The listing builds one solid part. Answer for the finished solid, in the listing's coordinates (mm). A direction names the side the tool comes from. Give positions to 0.01 mm unless a question says otherwise; leave off trailing zeros. Loops run counter-clockwise (first coordinate to the right, second up) from the corner with the lowest first, then second, coordinate; pieces in that order, holes last.
Item 1: Section B-B, the plane y = 7.25 is taken. Give the vertices of the cut face in (x, z).
Item 2: A tool of negligible diameter and unlimited length cuts with its end or side. For faces 4 (the face through (-4.33, 10.9, -3.16)), 5 (the face through (-7.81, 6.38, -1.73)), from which of +Z, -Z, +X, -X, +Y, -Y can it reach the whole face along a straight path? Write none if from no direction.
Item 3: Section A-A, the plane x = 0 is taken. Give the vertices of the cut face in (y, z).
Item 4: Each of these flat-tipped pins is pushed along its axis until it touches: pin 1 Ø3 at (y, z) = (10, -5) entering from -X; pin 2 Ø3 at (x, y) = (-6, 7) entering from -Z; pin 3 Ø6 at (x, y) = (-4, 11) entering from -Z. Where does it stop, or does it pass through?
Item 5: Consider line 1 along Y through (x, z) = (-0.25, -7); line 2 along Z through (x, y) = (-5.5, 11.25). Determine where each line is inside the solid, lowest interval first.
Item 6: The mould has two halves that part along Y. Classify faces 1 (the face through (-2, 5.9, 4)), 2 (the face through (-7.81, 15.51, -1.73)), 3 (the face through (0.01, 10.9, -5.36)): pulls with the +Y half, pulls with the -Y half, needs draft (parallel to the pull), parting line crosses it, or undercut.
from build123d import *
from OCP.BRepFilletAPI import BRepFilletAPI_MakeChamfer

# Parameters (mm, degrees)
SKETCH_1_R               = 8
SKETCH_1_R_2             = 2.5
EXTRUDE_1_DEPTH          = 7.45
SKETCH_2_R               = 2.5
EXTRUDE_2_DEPTH          = 7
SKETCH_3_R               = 8
SKETCH_3_R_2             = 2.5
EXTRUDE_3_DEPTH          = 1.55
CUT_EXTRUDE_1_REACH      = 21.596
CUT_EXTRUDE_1_END_RADIUS = 8
SKETCH_4_R               = 1.25
CUT_EXTRUDE_2_REACH      = 21.596
CUT_EXTRUDE_2_END_RADIUS = 8
SKETCH_5_R               = 1.25
CHAMFER_1_SIZE           = 1
CHAMFER_1_SIZE2          = 0.577350269
ESBO_O1_R                = 8
CORTE_EXTRUS_O1_DEPTH    = 5.9
ESBO_O2_R                = 4
CORTE_EXTRUS_O2_DEPTH    = 10.1


with BuildPart() as part:
    # Эскиз1 → Бобышка-Вытянуть1 (new body)
    with BuildSketch(Plane(origin=(0, 0, 0), x_dir=(1, 0, 0), z_dir=(0, 1, 0))):
        with Locations(Location((0, 0, 0), (0, 0, 270))):
            Circle(SKETCH_1_R)
        with Locations(Location((0, 0, 0), (0, 0, 270))):
            Circle(SKETCH_1_R_2, mode=Mode.SUBTRACT)
    extrude(amount=EXTRUDE_1_DEPTH)

    # Эскиз2 → Бобышка-Вытянуть2 (add)
    with BuildSketch(Plane(origin=(0, 7.45, 0), x_dir=(1, 0, 0), z_dir=(0, 1, 0))):
        with BuildLine():
            ThreePointArc((-2.557469435, 5.549004423), (-2.773881953, 5.444049863), (-2.985996064, 5.3306592))
            ThreePointArc((-2.985996064, 5.3306592), (-3.059404709, 5.231014138), (-3.032930262, 5.110113057))
            ThreePointArc((-3.032930262, 5.110113057), (-3.150528952, 4.33633109), (-3.922779328, 4.463599867))
            ThreePointArc((-3.922779328, 4.463599867), (-4.029582035, 4.526139051), (-4.14703464, 4.487115298))
            ThreePointArc((-4.14703464, 4.487115298), (-4.320422433, 4.320422433), (-4.487115298, 4.14703464))
            ThreePointArc((-4.487115298, 4.14703464), (-4.526139051, 4.029582035), (-4.463599867, 3.922779328))
            ThreePointArc((-4.463599867, 3.922779328), (-4.33633109, 3.150528952), (-5.110113057, 3.032930262))
            ThreePointArc((-5.110113057, 3.032930262), (-5.231014138, 3.059404709), (-5.3306592, 2.985996064))
            ThreePointArc((-5.3306592, 2.985996064), (-5.444049863, 2.773881953), (-5.549004423, 2.557469435))
            ThreePointArc((-5.549004423, 2.557469435), (-5.549823367, 2.433706366), (-5.457341217, 2.351456627))
            ThreePointArc((-5.457341217, 2.351456627), (-5.097662927, 1.65633109), (-5.797233315, 1.305376312))
            ThreePointArc((-5.797233315, 1.305376312), (-5.92039813, 1.293194518), (-5.992481697, 1.19258673))
            ThreePointArc((-5.992481697, 1.19258673), (-6.034775761, 0.955814581), (-6.067718334, 0.717561302))
            ThreePointArc((-6.067718334, 0.717561302), (-6.030252304, 0.599602562), (-5.916879985, 0.549956967))
            ThreePointArc((-5.916879985, 0.549956967), (-5.36, 0), (-5.916879985, -0.549956967))
            ThreePointArc((-5.916879985, -0.549956967), (-6.030252304, -0.599602562), (-6.067718334, -0.717561302))
            ThreePointArc((-6.067718334, -0.717561302), (-6.034775761, -0.955814581), (-5.992481697, -1.19258673))
            ThreePointArc((-5.992481697, -1.19258673), (-5.92039813, -1.293194518), (-5.797233315, -1.305376312))
            ThreePointArc((-5.797233315, -1.305376312), (-5.097662927, -1.65633109), (-5.457341217, -2.351456627))
            ThreePointArc((-5.457341217, -2.351456627), (-5.549823367, -2.433706366), (-5.549004423, -2.557469435))
            ThreePointArc((-5.549004423, -2.557469435), (-5.444049863, -2.773881953), (-5.3306592, -2.985996064))
            ThreePointArc((-5.3306592, -2.985996064), (-5.231014138, -3.059404709), (-5.110113057, -3.032930262))
            ThreePointArc((-5.110113057, -3.032930262), (-4.33633109, -3.150528952), (-4.463599867, -3.922779328))
            ThreePointArc((-4.463599867, -3.922779328), (-4.526139051, -4.029582035), (-4.487115298, -4.14703464))
            ThreePointArc((-4.487115298, -4.14703464), (-4.320422433, -4.320422433), (-4.14703464, -4.487115298))
            ThreePointArc((-4.14703464, -4.487115298), (-4.029582035, -4.526139051), (-3.922779328, -4.463599867))
            ThreePointArc((-3.922779328, -4.463599867), (-3.150528952, -4.33633109), (-3.032930262, -5.110113057))
            ThreePointArc((-3.032930262, -5.110113057), (-3.059404709, -5.231014138), (-2.985996064, -5.3306592))
            ThreePointArc((-2.985996064, -5.3306592), (-2.773881953, -5.444049863), (-2.557469435, -5.549004423))
            ThreePointArc((-2.557469435, -5.549004423), (-2.433706366, -5.549823367), (-2.351456627, -5.457341217))
            ThreePointArc((-2.351456627, -5.457341217), (-1.65633109, -5.097662927), (-1.305376312, -5.797233315))
            ThreePointArc((-1.305376312, -5.797233315), (-1.293194518, -5.92039813), (-1.19258673, -5.992481697))
            ThreePointArc((-1.19258673, -5.992481697), (-0.955814581, -6.034775761), (-0.717561302, -6.067718334))
            ThreePointArc((-0.717561302, -6.067718334), (-0.599602562, -6.030252304), (-0.549956967, -5.916879985))
            ThreePointArc((-0.549956967, -5.916879985), (0, -5.36), (0.549956967, -5.916879985))
            ThreePointArc((0.549956967, -5.916879985), (0.599602562, -6.030252304), (0.717561302, -6.067718334))
            ThreePointArc((0.717561302, -6.067718334), (0.955814581, -6.034775761), (1.19258673, -5.992481697))
            ThreePointArc((1.19258673, -5.992481697), (1.293194518, -5.92039813), (1.305376312, -5.797233315))
            ThreePointArc((1.305376312, -5.797233315), (1.65633109, -5.097662927), (2.351456627, -5.457341217))
            ThreePointArc((2.351456627, -5.457341217), (2.433706366, -5.549823367), (2.557469435, -5.549004423))
            ThreePointArc((2.557469435, -5.549004423), (2.773881953, -5.444049863), (2.985996064, -5.3306592))
            ThreePointArc((2.985996064, -5.3306592), (3.059404709, -5.231014138), (3.032930262, -5.110113057))
            ThreePointArc((3.032930262, -5.110113057), (3.150528952, -4.33633109), (3.922779328, -4.463599867))
            ThreePointArc((3.922779328, -4.463599867), (4.029582035, -4.526139051), (4.14703464, -4.487115298))
            ThreePointArc((4.14703464, -4.487115298), (4.320422433, -4.320422433), (4.487115298, -4.14703464))
            ThreePointArc((4.487115298, -4.14703464), (4.526139051, -4.029582035), (4.463599867, -3.922779328))
            ThreePointArc((4.463599867, -3.922779328), (4.33633109, -3.150528952), (5.110113057, -3.032930262))
            ThreePointArc((5.110113057, -3.032930262), (5.231014138, -3.059404709), (5.3306592, -2.985996064))
            ThreePointArc((5.3306592, -2.985996064), (5.444049863, -2.773881953), (5.549004423, -2.557469435))
            ThreePointArc((5.549004423, -2.557469435), (5.549823367, -2.433706366), (5.457341217, -2.351456627))
            ThreePointArc((5.457341217, -2.351456627), (5.097662927, -1.65633109), (5.797233315, -1.305376312))
            ThreePointArc((5.797233315, -1.305376312), (5.92039813, -1.293194518), (5.992481697, -1.19258673))
            ThreePointArc((5.992481697, -1.19258673), (6.034775761, -0.955814581), (6.067718334, -0.717561302))
            ThreePointArc((6.067718334, -0.717561302), (6.030252304, -0.599602562), (5.916879985, -0.549956967))
            ThreePointArc((5.916879985, -0.549956967), (5.36, 0), (5.916879985, 0.549956967))
            ThreePointArc((5.916879985, 0.549956967), (6.030252304, 0.599602562), (6.067718334, 0.717561302))
            ThreePointArc((6.067718334, 0.717561302), (6.034775761, 0.955814581), (5.992481697, 1.19258673))
            ThreePointArc((5.992481697, 1.19258673), (5.92039813, 1.293194518), (5.797233315, 1.305376312))
            ThreePointArc((5.797233315, 1.305376312), (5.097662927, 1.65633109), (5.457341217, 2.351456627))
            ThreePointArc((5.457341217, 2.351456627), (5.549823367, 2.433706366), (5.549004423, 2.557469435))
            ThreePointArc((5.549004423, 2.557469435), (5.444049863, 2.773881953), (5.3306592, 2.985996064))
            ThreePointArc((5.3306592, 2.985996064), (5.231014138, 3.059404709), (5.110113057, 3.032930262))
            ThreePointArc((5.110113057, 3.032930262), (4.33633109, 3.150528952), (4.463599867, 3.922779328))
            ThreePointArc((4.463599867, 3.922779328), (4.526139051, 4.029582035), (4.487115298, 4.14703464))
            ThreePointArc((4.487115298, 4.14703464), (4.320422433, 4.320422433), (4.14703464, 4.487115298))
            ThreePointArc((4.14703464, 4.487115298), (4.029582035, 4.526139051), (3.922779328, 4.463599867))
            ThreePointArc((3.922779328, 4.463599867), (3.150528952, 4.33633109), (3.032930262, 5.110113057))
            ThreePointArc((3.032930262, 5.110113057), (3.059404709, 5.231014138), (2.985996064, 5.3306592))
            ThreePointArc((2.985996064, 5.3306592), (2.773881953, 5.444049863), (2.557469435, 5.549004423))
            ThreePointArc((2.557469435, 5.549004423), (2.433706366, 5.549823367), (2.351456627, 5.457341217))
            ThreePointArc((2.351456627, 5.457341217), (1.65633109, 5.097662927), (1.305376312, 5.797233315))
            ThreePointArc((1.305376312, 5.797233315), (1.293194518, 5.92039813), (1.19258673, 5.992481697))
            ThreePointArc((1.19258673, 5.992481697), (0.955814581, 6.034775761), (0.717561302, 6.067718334))
            ThreePointArc((0.717561302, 6.067718334), (0.599602562, 6.030252304), (0.549956967, 5.916879985))
            ThreePointArc((0.549956967, 5.916879985), (0, 5.36), (-0.549956967, 5.916879985))
            ThreePointArc((-0.549956967, 5.916879985), (-0.599602562, 6.030252304), (-0.717561302, 6.067718334))
            ThreePointArc((-0.717561302, 6.067718334), (-0.955814581, 6.034775761), (-1.19258673, 5.992481697))
            ThreePointArc((-1.19258673, 5.992481697), (-1.293194518, 5.92039813), (-1.305376312, 5.797233315))
            ThreePointArc((-1.305376312, 5.797233315), (-1.65633109, 5.097662927), (-2.351456627, 5.457341217))
            ThreePointArc((-2.351456627, 5.457341217), (-2.433706366, 5.549823367), (-2.557469435, 5.549004423))
        make_face()
        with Locations(Location((0, 0, 0), (0, 0, 270))):
            Circle(SKETCH_2_R, mode=Mode.SUBTRACT)
    extrude(amount=EXTRUDE_2_DEPTH)

    # Эскиз3 → Бобышка-Вытянуть3 (add)
    with BuildSketch(Plane(origin=(0, 14.45, 0), x_dir=(1, 0, 0), z_dir=(0, 1, 0))):
        with Locations(Location((0, 0, 0), (0, 0, 270))):
            Circle(SKETCH_3_R)
        with Locations(Location((0, 0, 0), (0, 0, 270))):
            Circle(SKETCH_3_R_2, mode=Mode.SUBTRACT)
    extrude(amount=EXTRUDE_3_DEPTH)

    # Вырез-Вытянуть1: up to this cylinder (the profile starts inside it)
    cut_extrude_1_end = Plane(origin=(0, 3.725, 0), z_dir=(0, -1, 0)) * Cylinder(CUT_EXTRUDE_1_END_RADIUS, 60.192, mode=Mode.PRIVATE)
    # Эскиз4 → Вырез-Вытянуть1 (cut, up to the surface)
    with BuildSketch(Plane.XY, mode=Mode.PRIVATE) as cut_extrude_1_sk1:
        with Locations(Location((0, 3.725, 0), (0, 0, 180))):
            Circle(SKETCH_4_R)
    cut_extrude_1_tool1 = extrude(cut_extrude_1_sk1.sketch, amount=CUT_EXTRUDE_1_REACH, mode=Mode.PRIVATE) & cut_extrude_1_end
    add(cut_extrude_1_tool1.solids().sort_by_distance((0, 3.725, 0))[0], mode=Mode.SUBTRACT)

    # Вырез-Вытянуть2: up to this cylinder (the profile starts inside it)
    cut_extrude_2_end = Plane(origin=(0, 3.725, 0), z_dir=(0, -1, 0)) * Cylinder(CUT_EXTRUDE_2_END_RADIUS, 60.192, mode=Mode.PRIVATE)
    # Эскиз5 → Вырез-Вытянуть2 (cut, up to the surface)
    with BuildSketch(Plane(origin=(0, 0, 0), x_dir=(0, 0, -1), z_dir=(1, 0, 0)), mode=Mode.PRIVATE) as cut_extrude_2_sk1:
        with Locations(Location((0, 3.725, 0), (0, 0, 180))):
            Circle(SKETCH_5_R)
    cut_extrude_2_tool1 = extrude(cut_extrude_2_sk1.sketch, amount=CUT_EXTRUDE_2_REACH, mode=Mode.PRIVATE) & cut_extrude_2_end
    add(cut_extrude_2_tool1.solids().sort_by_distance((0, 3.725, 0))[0], mode=Mode.SUBTRACT)

    # Фаска1: one chamfer whose edges measure the first distance from different faces: ONE call of the kernel's chamfer builder (chamfer() names one face for all edges)
    chamfer_1_edges_1 = [part.edges().sort_by_distance(p)[0] for p in [
        (0, 14.45, -8),
    ]]
    chamfer_1_side_1 = [part.faces().sort_by_distance(p)[0] for p in [
        (0, 14.45, -7.77372583),
    ]]
    chamfer_1_edges_2 = [part.edges().sort_by_distance(p)[0] for p in [
        (0, 7.45, -8),
    ]]
    chamfer_1_side_2 = [part.faces().sort_by_distance(p)[0] for p in [
        (0, 7.45, -7.77372583),
    ]]
    chamfer_1 = BRepFilletAPI_MakeChamfer(part.part.solid().wrapped)
    for e in chamfer_1_edges_1:
        chamfer_1.Add(CHAMFER_1_SIZE, CHAMFER_1_SIZE2, e.wrapped, chamfer_1_side_1[0].wrapped)  # the first distance lies on this face
    for e in chamfer_1_edges_2:
        chamfer_1.Add(CHAMFER_1_SIZE, CHAMFER_1_SIZE2, e.wrapped, chamfer_1_side_2[0].wrapped)  # the first distance lies on this face
    add(Compound.cast(chamfer_1.Shape()), mode=Mode.REPLACE)

    # Esboço1 → Corte-extrusão1 (cut)
    with BuildSketch(Plane.XZ):
        with Locations(Location((0, 0, 0), (0, 0, 270))):
            Circle(ESBO_O1_R)
    extrude(amount=-CORTE_EXTRUS_O1_DEPTH, mode=Mode.SUBTRACT)

    # Esboço2 → Corte-extrusão2 (cut)
    with BuildSketch(Plane(origin=(0, 16, 0), x_dir=(1, 0, 0), z_dir=(0, 1, 0))):
        with Locations(Location((0, 0, 0), (0, 0, 270))):
            Circle(ESBO_O2_R)
    extrude(amount=-CORTE_EXTRUS_O2_DEPTH, mode=Mode.SUBTRACT)


solid = part.part
Worked answers:
1. outline: circle Ø14.69 at (0, 0); hole circle Ø8 at (0, 0)
2. face 4: none
2. face 5: +Y, -Y
3. outline: (5.9, -8) - (6.87, -8) - (7.45, -7) - (7.45, -5.36) - (14.45, -5.36) - (14.45, -7) - (15.03, -8) - (16, -8) - (16, -4) - (5.9, -4) - close; (5.9, 4) - (16, 4) - (16, 8) - (15.03, 8) - (14.45, 7) - (14.45, 5.36) - (7.45, 5.36) - (7.45, 7) - (6.87, 8) - (5.9, 8) - close
4. pin 1: stops at x = -4.53
4. pin 2: stops at z = -6.61
4. pin 3: stops at z = -6.03
5. line 1: y = 5.9 to 7.45, 14.45 to 16
5. line 2: z = -2.66 to -2.37, -1.29 to -0.37, 0.37 to 1.29, 2.37 to 2.66
6. face 1: pulls with the -Y half
6. face 2: needs draft
6. face 3: undercut
